Geometry check sheet. Reference: the model listing, model coordinates, mm. Round coordinates to 2 decimals unless told otherwise and drop trailing zeros. Order: outer loops, then holes, each group sorted by start corner. A loop starts at its lowest first (then second) coordinate and runs counter-clockwise, first axis right, second up. Notation, with made-up numbers: (30, -17) - (86, -17) arc R24 cw to (86, 15) - close; hole circle Ø5 at (10, -17.5). An arc over 180 degrees is marked (long way). Return JSON: item names as keys, results as strings. Group by question number.
Q1. Gauge pin test, flat end, axial feed: pin 1 Ø12 at (x, y) = (-11, 56.5) entering from -Z. Record the tip position at first contact, or that the pin passes through.
Q2. Material ranges on line 1 along Y through (x, z) = (0, 1.25); line 2 along X through (y, z) = (-90.17, 1.7); line 3 along Y through (x, z) = (1, 0.25), recorded low to high.
Q3. Sectioned sample at A-A, the plane y = 25.4. Record the cut outline in (x, z), then the cut area to 3 significant figures.
Q4. Draft check along Y on faces 1 (the cylindrical face through (-0.33, 27.88, 1.29)), 2 (the flat face through (0, 2, 2.54)). Enter one of: pulls with the +Y half, pulls with the -Y half, needs draft (parallel to the pull), parting line crosses it, or undercut.
```python
from build123d import *

# Parameters (mm, degrees)
SKETCH1_W           = 38.862
SKETCH1_H           = 228.6
BOSS_EXTRUDE1_DEPTH = 2.54
SKETCH2_R           = 1.5875
CUT_EXTRUDE1_DEPTH  = 116.967691022
SKETCH3_R           = 2.5
CUT_EXTRUDE2_DEPTH  = 5.08
SKETCH4_W           = 38.862
SKETCH4_H           = 2.54
CUT_EXTRUDE3_DEPTH  = 116.967691022


with BuildPart() as part:
    # Sketch1 → Boss-Extrude1 (new body)
    with BuildSketch(Plane.XY):
        Rectangle(SKETCH1_W, SKETCH1_H)
    extrude(amount=BOSS_EXTRUDE1_DEPTH)

    # Sketch2 → Cut-Extrude1 (cut, through all)
    with BuildSketch(Plane.XY.offset(2.54)):
        with Locations((0, -90.17)):
            Circle(SKETCH2_R)
    cut_extrude1 = extrude(amount=-CUT_EXTRUDE1_DEPTH, mode=Mode.SUBTRACT)

    # Mirror1: Cut-Extrude1 across plane
    add(cut_extrude1.mirror(Plane.ZX), mode=Mode.SUBTRACT)

    # Sketch3 → Cut-Extrude2 (cut)
    with BuildSketch(Plane.XY.offset(2.54)):
        with Locations((0, -25.4)):
            Circle(SKETCH3_R)
        with Locations((0, 25.4)):
            Circle(SKETCH3_R)
    extrude(amount=-CUT_EXTRUDE2_DEPTH, mode=Mode.SUBTRACT)

    # Sketch4 → Cut-Extrude3 (cut, through all)
    with BuildSketch(Plane.XY.offset(2.54)):
        with Locations((0, 113.03)):
            Rectangle(SKETCH4_W, SKETCH4_H)
        with Locations((0, -113.03)):
            Rectangle(SKETCH4_W, SKETCH4_H)
    extrude(amount=-CUT_EXTRUDE3_DEPTH, mode=Mode.SUBTRACT)


solid = part.part
```
Reply:
{
 "1": {"pin 1": "z = 0"},
 "2": {"line 1": "-111.76 to -91.76, -88.58 to -27.9, -22.9 to 22.9, 27.9 to 88.58, 91.76 to 111.76", "line 2": "-19.43 to -1.59, 1.59 to 19.43", "line 3": "-111.76 to -91.4, -88.94 to -27.69, -23.11 to 23.11, 27.69 to 88.94, 91.4 to 111.76"},
 "3": {"outline": "(-19.43, 0) - (-2.5, 0) - (-2.5, 2.54) - (-19.43, 2.54) - close; (2.5, 0) - (19.43, 0) - (19.43, 2.54) - (2.5, 2.54) - close", "area": "86.0 mm^2"},
 "4": {"face 1": "undercut", "face 2": "needs draft"}
}
